The listing builds one solid part. Answer for the finished solid, in the listing's coordinates (mm). A direction names the side the tool comes from. Coordinates: 2 decimals unless noted, no trailing zeros. Order: outer loops, then holes, each group sorted by start corner. A loop starts at its lowest first (then second) coordinate and runs counter-clockwise, first axis right, second up. Notation, with made-up numbers: (-7.5, -7) - (8.5, -7) arc R14 cw to (8.5, 15) - close; hole circle Ø7 at (56, 80). An arc over 180 degrees is marked (long way). Use a Markdown table: item, result. Add a question column.
Item 1: The part is cut by section A-A, the plane z = 29. Give the vertices of the cut face in (x, y).
Item 2: For faces 1 (the flat face through (25, -19.05, 26)), 2 (the cylindrical face through (42.64, -3.38, 8.26)), 3 (the flat face through (38, -25.4, 38)), determine the directions among +Z, -Z, +X, -X, +Y, -Y from which every point of the face is accessible in a straight line to the end or side of a thin tool.
Item 3: The part is cut by section C-C, the plane x = 21. Give the vertices of the cut face in (y, z), then the cut area to 3 significant figures.
Item 4: Find the intervals of material crossed by line 1 along Z through (x, y) = (18, -1.75); line 2 along Y through (x, z) = (7, 36); line 3 along Y through (x, z) = (45, 27.5), in increasing order.
Item 5: The part is cut by section B-B, the plane y = -4.25. Give the vertices of the cut face in (x, z).
Item 6: Flat-ended cylindrical pins translate along their axes: P1, Ø1, axis at x = 28.5, z = 22, coming from the +Y side; P2, Ø2, axis at x = 45.5, z = 19.5, coming from the -Y side. Find the tip coordinate at first contact, or state that the pin passes through.
Item 7: The part is cut by section D-D, the plane y = -21.25. Give the vertices of the cut face in (x, z), then the cut area to 3 significant figures.
Item 8: The mould has two halves that part along X. Classify faces 4 (the cylindrical face through (8.16, -3.38, 42.54)), 5 (the flat face through (25, -3, 44.45)), 6 (the flat face through (25, -9, 50.8)), 7 (the flat face through (50.8, -9, 25)): released by +X, released by -X, zero draft, split by the parting line, or undercut.
from build123d import *

# Parameters (mm, degrees)
F0_W     = 50.8
F0_H     = 50.8
F1_DEPTH = 19.05
F2_R     = 6.35
F3_DEPTH = 6.35
F5_DEPTH = 6.858


with BuildPart() as f1:
    # F0 (on Front) → F1 (new body)
    with BuildSketch(Plane.XZ):
        with Locations((25.4, 25.4)):
            Rectangle(F0_W, F0_H)
    extrude(amount=F1_DEPTH)

    # F2 (on face) → F3 (join)
    with BuildSketch(Plane.XZ.offset(19.05)):
        with Locations((12.7, 38.1)):
            Circle(F2_R)
        with Locations((38.1, 38.1)):
            Circle(F2_R)
        with Locations((12.7, 12.7)):
            Circle(F2_R)
        with Locations((38.1, 12.7)):
            Circle(F2_R)
    extrude(amount=F3_DEPTH)

    # F4 (on face) → F5 (cut)
    with BuildSketch(Plane(origin=(0, 0, 0), x_dir=(-1, 0, 0), z_dir=(0, 1, 0))):
        with BuildLine():
            Line((-12.7, 44.45), (-38.1, 44.45))
            ThreePointArc((-38.1, 44.45), (-42.590128, 42.590128), (-44.45, 38.1))
            Line((-44.45, 38.1), (-44.45, 12.7))
            ThreePointArc((-44.45, 12.7), (-42.590128, 8.209872), (-38.1, 6.35))
            Line((-38.1, 6.35), (-12.7, 6.35))
            ThreePointArc((-12.7, 6.35), (-8.209872, 8.209872), (-6.35, 12.7))
            Line((-6.35, 12.7), (-6.35, 38.1))
            ThreePointArc((-6.35, 38.1), (-8.209872, 42.590128), (-12.7, 44.45))
        make_face()
    extrude(amount=-F5_DEPTH, mode=Mode.SUBTRACT)


solid = f1.part
Solution:
| question | item | result |
|---|---|---|
| 1 | outline | (0, -19.05) - (50.8, -19.05) - (50.8, 0) - (44.45, 0) - (44.45, -6.86) - (6.35, -6.86) - (6.35, 0) - (0, 0) - close |
| 2 | face 1 | -Y |
| 2 | face 2 | +Y |
| 2 | face 3 | +Z, -Z, +X, -X, -Y |
| 3 | outline | (-19.05, 0) - (0, 0) - (0, 6.35) - (-6.86, 6.35) - (-6.86, 44.45) - (0, 44.45) - (0, 50.8) - (-19.05, 50.8) - close |
| 3 | area | 706 mm2 |
| 4 | line 1 | z = 0 to 6.35, 44.45 to 50.8 |
| 4 | line 2 | y = -25.4 to -6.86 |
| 4 | line 3 | y = -19.05 to 0 |
| 5 | outline | (0, 0) - (50.8, 0) - (50.8, 50.8) - (0, 50.8) - close; hole (6.35, 12.7) arc R6.35 ccw to (12.7, 6.35) - (38.1, 6.35) arc R6.35 ccw to (44.45, 12.7) - (44.45, 38.1) arc R6.35 ccw to (38.1, 44.45) - (12.7, 44.45) arc R6.35 ccw to (6.35, 38.1) - close |
| 6 | P1 | stops at y = -6.86 |
| 6 | P2 | stops at y = -19.05 |
| 7 | outline | circle Ø12.7 at (12.7, 12.7); circle Ø12.7 at (12.7, 38.1); circle Ø12.7 at (38.1, 12.7); circle Ø12.7 at (38.1, 38.1) |
| 7 | area | 507 mm2 |
| 8 | face 4 | undercut |
| 8 | face 5 | undercut |
| 8 | face 6 | zero draft |
| 8 | face 7 | released by +X |
